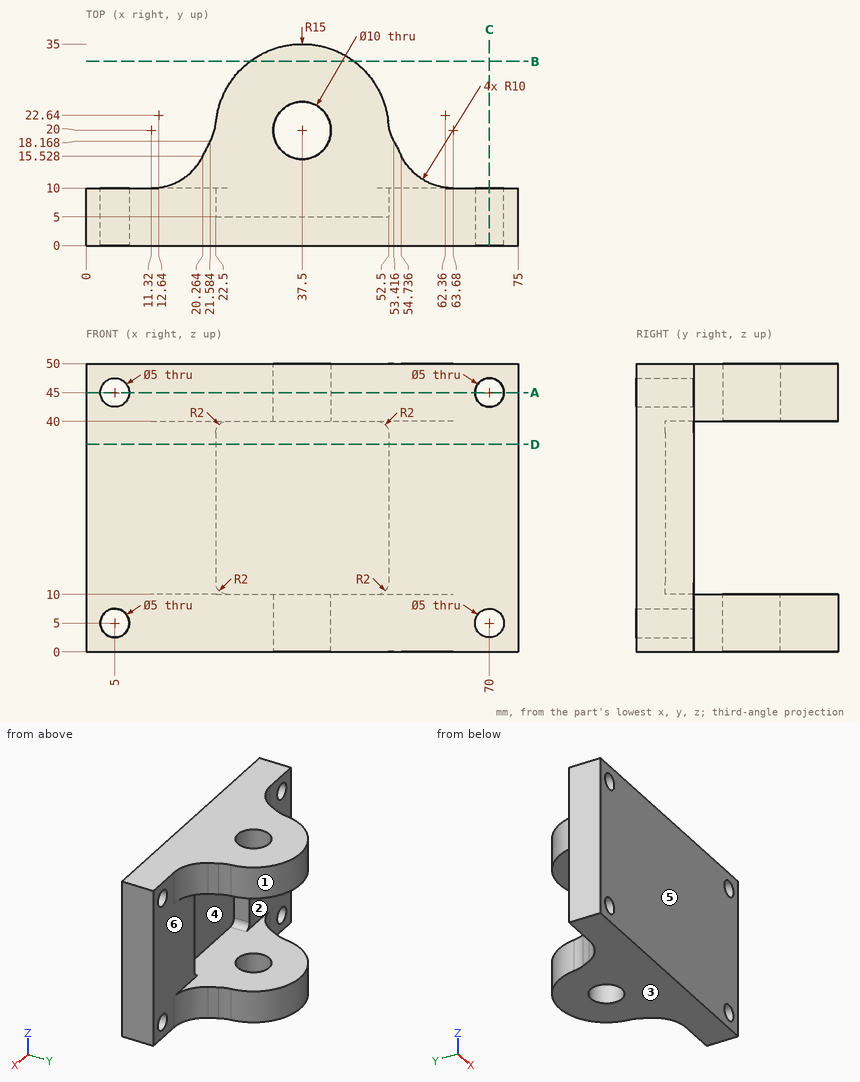
Geometry: see drawing. Coordinates: mm, zero at the bounding-box minimum. A direction names the side the tool comes from. Coordinates: 2 decimals unless noted, no trailing zeros. Loops run counter-clockwise (first coordinate to the right, second up) from the corner with the lowest first, then second, coordinate; pieces in that order, holes last.
(1) First-contact query: pin 1 Ø7.5 at (x, z) = (17, 15.5) entering from +Y; pin 2 Ø4.5 at (x, z) = (70, 5) entering from +Y; pin 3 Ø1 at (y, z) = (25, 41.5) entering from +X; pin 4 Ø15 at (x, z) = (33, 19) entering from +Y. Flat tips, straight axial feed; report the tip coordinate or a pass-through.
(2) Section A-A on z = 45. Return the cut outline in (x, y), then the cut area to 3 significant figures.
(3) Section B-B on y = 32. Return the cut outline in (x, z), then the cut area to 3 significant figures.
(4) Pull-direction query (Z, two-part tool) for the marked faces 1, 2 and 3; classes: released by +Z, released by -Z, zero draft, split by the parting line, or undercut.
(5) Section C-C on x = 70. Return the cut outline in (y, z).
(6) Material intervals for probe 1 along X at (y, z) = (3, 45); probe 2 along Z at (x, y) = (5, 6); probe 3 along Y at (x, z) = (37.5, 47), sorted ascending.
(7) Section D-D on z = 36. Return the cut outline in (x, y), then the cut area to 3 significant figures.
(8) Set-up query: the marked faces 4, 5 and 6. Return all of +Z, -Z, +X, -X, +Y, -Y with unobstructed straight access to the full face (end or side cutting, diameter ignored); none if empty.
Data:
1. pin 1: stops at y = 10
1. pin 2: passes through
1. pin 3: stops at x = 51.81
1. pin 4: stops at y = 5
2. outline: (0, 0) - (2.5, 0) - (2.5, 10) - (0, 10) - close; (7.5, 0) - (67.5, 0) - (67.5, 10) - (63.68, 10) arc R10 cw to (54.74, 15.53) - (53.42, 18.17) arc R10 cw to (52.42, 21.58) arc R15 ccw to (22.58, 21.58) arc R10 cw to (21.58, 18.17) - (20.26, 15.53) arc R10 cw to (11.32, 10) - (7.5, 10) - close; (72.5, 0) - (75, 0) - (75, 10) - (72.5, 10) - close; hole circle Ø10 at (37.5, 20)
2. area: 1,290 mm2
3. outline: (28.5, 0) - (46.5, 0) - (46.5, 10) - (28.5, 10) - close; (28.5, 40) - (46.5, 40) - (46.5, 50) - (28.5, 50) - close
3. area: 360 mm2
4. face 1: zero draft
4. face 2: undercut
4. face 3: released by -Z
5. outline: (0, 0) - (10, 0) - (10, 2.5) - (0, 2.5) - close; (0, 7.5) - (10, 7.5) - (10, 42.5) - (0, 42.5) - close; (0, 47.5) - (10, 47.5) - (10, 50) - (0, 50) - close
6. probe 1: x = 0 to 2.5, 7.5 to 67.5, 72.5 to 75
6. probe 2: z = 0 to 2.5, 7.5 to 42.5, 47.5 to 50
6. probe 3: y = 0 to 15, 25 to 35
7. outline: (0, 0) - (75, 0) - (75, 10) - (52.5, 10) - (52.5, 5) - (22.5, 5) - (22.5, 10) - (0, 10) - close
7. area: 600 mm2
8. face 4: +Y
8. face 5: +Z, -Z, +X, -X, -Y
8. face 6: +X, +Y
